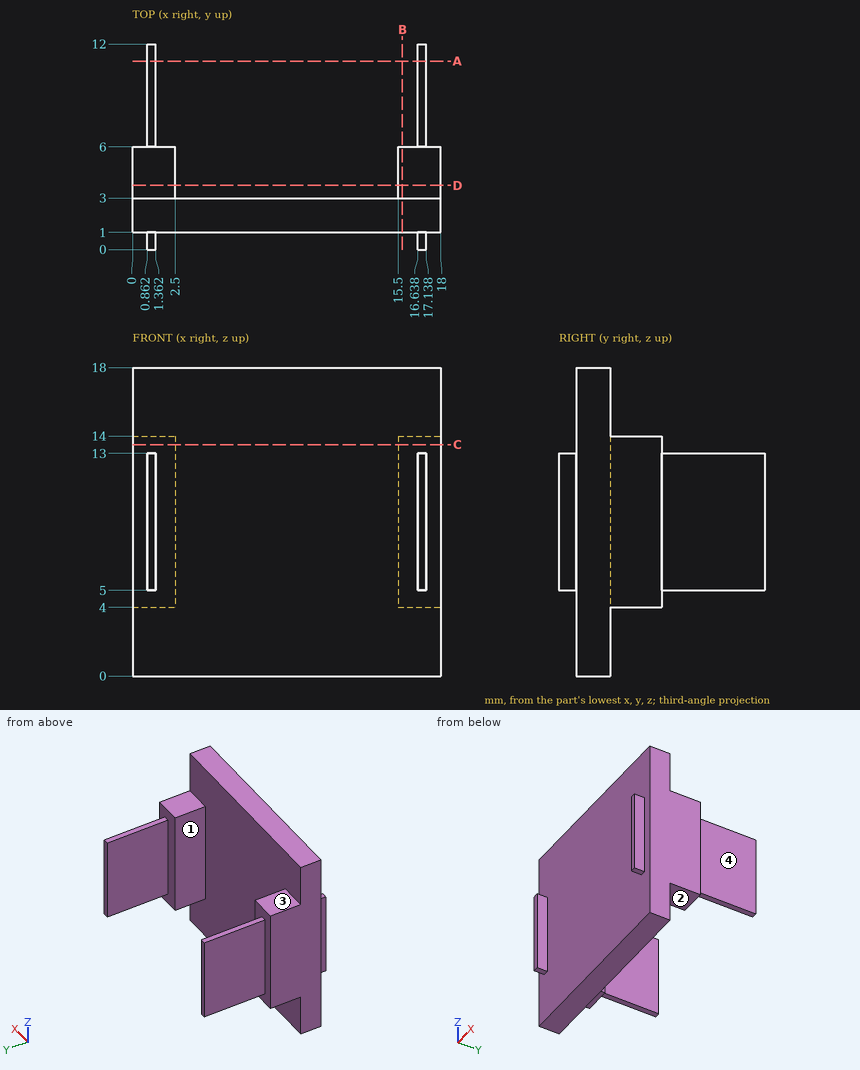
Print and shaded views of the part. All mm, measured from the part's lowest x, y and z. A direction names the side the tool comes from. Coordinates: 2 decimals unless noted, no trailing zeros. Write each loop counter-clockwise with the first axis right and the second up, starting at its lowest first coordinate (ties: lowest second). Pieces come first, ordered by that corner, then holes.
(1) Cut at D-D, the plane y = 3.75. List the corners of the cut face in (x, z), and give its area (3 significant figures).
(2) Cut at A-A, the plane y = 11. List the corners of the cut face in (x, z).
(3) Cut at C-C, the plane z = 13.5. List the corners of the cut face in (x, y), and give its area (3 significant figures).
(4) Flat gauge pins, fed straight in: pin 1 (5.5 mm diameter, centred on x = 10.5, z = 5, fed in from -Y); pin 2 (0.8 mm diameter, centred on y = 0.5, z = 8.5, fed in from +X); pin 3 (8 mm diameter, centred on x = 7.5, z = 11, fed in from +Y); pin 4 (1 mm diameter, centred on x = 8, y = 4, fed in from -Z). Where does each tip first touch, or does it go through?
(5) 3-axis set-ups, long thin cutter, end or side, ignore diameter. For the marked faces 1, 2, 3 and 4: which of +Z, -Z, +X, -X, +Y, -Y reach the whole face in a straight line?
(6) Cut at B-B, the plane x = 15.75. List the corners of the cut face in (y, z).
(7) Drill centre lines: probe 1 along X at (y, z) = (4, 12.75); probe 2 along X at (y, z) = (7, 8); probe 3 along Y at (x, z) = (9.75, 3). Where is each one in solid material? Low to high.
Geometry says:
1. outline: (0, 4) - (2.5, 4) - (2.5, 14) - (0, 14) - close; (15.5, 4) - (18, 4) - (18, 14) - (15.5, 14) - close
1. area: 50.0 mm2
2. outline: (0.86, 5) - (1.36, 5) - (1.36, 13) - (0.86, 13) - close; (16.64, 5) - (17.14, 5) - (17.14, 13) - (16.64, 13) - close
3. outline: (0, 1) - (18, 1) - (18, 6) - (15.5, 6) - (15.5, 3) - (2.5, 3) - (2.5, 6) - (0, 6) - close
3. area: 51.0 mm2
4. pin 1: stops at y = 1
4. pin 2: stops at x = 17.14
4. pin 3: stops at y = 3
4. pin 4: passes through
5. face 1: +Z, -Z, +Y
5. face 2: -Z, +X, -X, +Y
5. face 3: +Z, +X, -X, +Y
5. face 4: +Z, -Z, +X, +Y
6. outline: (1, 0) - (3, 0) - (3, 4) - (6, 4) - (6, 14) - (3, 14) - (3, 18) - (1, 18) - close
7. probe 1: x = 0 to 2.5, 15.5 to 18
7. probe 2: x = 0.86 to 1.36, 16.64 to 17.14
7. probe 3: y = 1 to 3
